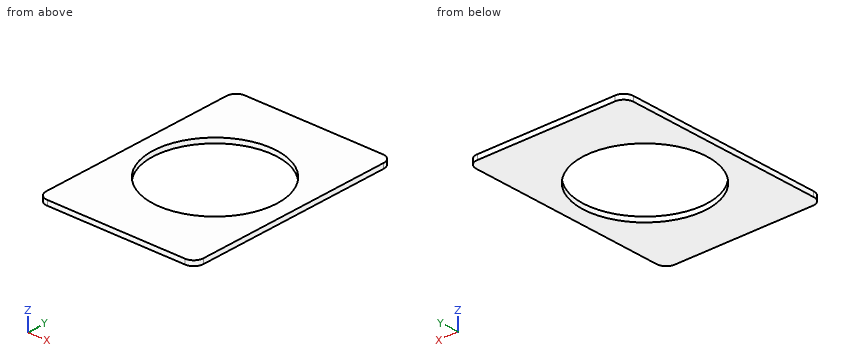
from build123d import *

# Parameters (mm, degrees)
F0_R     = 25
F1_DEPTH = 2


with BuildPart() as f1:
    # F0 (on Top) → F1 (new body)
    with BuildSketch(Plane.XY):
        with BuildLine():
            Line((31.70578804, -40.5199971151), (31.70578804, 40.5199971151))
            add(Edge.make_bspline(
                [(27.8376818991, 44.388103256), (29.9651402766, 44.388103256), (31.70578804, 42.6474554926), (31.70578804, 40.5199971151)],
                knots=[0, 0, 0, 0, 1, 1, 1, 1], degree=3))
            Line((27.8376818991, 44.388103256), (-27.8373296126, 44.388103256))
            add(Edge.make_bspline(
                [(-31.70578804, 40.5199971151), (-31.70578804, 42.6474554926), (-29.9651402766, 44.388103256), (-27.8373296126, 44.388103256)],
                knots=[0, 0, 0, 0, 1, 1, 1, 1], degree=3))
            Line((-31.70578804, 40.5199971151), (-31.70578804, -40.5199971151))
            add(Edge.make_bspline(
                [(-27.8373296126, -44.388103256), (-29.9651402766, -44.388103256), (-31.70578804, -42.6474554926), (-31.70578804, -40.5199971151)],
                knots=[0, 0, 0, 0, 1, 1, 1, 1], degree=3))
            Line((-27.8373296126, -44.388103256), (27.8376818991, -44.388103256))
            add(Edge.make_bspline(
                [(31.70578804, -40.5199971151), (31.70578804, -42.6474554926), (29.9651402766, -44.388103256), (27.8376818991, -44.388103256)],
                knots=[0, 0, 0, 0, 1, 1, 1, 1], degree=3))
        make_face()
        Circle(F0_R, mode=Mode.SUBTRACT)
    extrude(amount=F1_DEPTH)


solid = f1.part
CAD build for the part. Positions are in the model's coordinates, mm. Give positions to 0.01 mm unless a question says otherwise; leave off trailing zeros. Order: outer loops, then holes, each group sorted by start corner. A loop starts at its lowest first (then second) coordinate and runs counter-clockwise, first axis right, second up. Notation, with made-up numbers: (12, -34.75) - (22, -34.75) arc R7 ccw to (22, -24.75) - close; hole circle Ø5 at (8, 39). An arc over 180 degrees is marked (long way). Write each question's results on one line, items separated by ' | '.
1. Probe L1, parallel to Y at x = 0, z = 1.45; L2, parallel to X at y = 20, z = 1.8; L3, parallel to Y at x = 9.5, z = 0.55. List the from-to ranges inside material, lowest first. Write a range as from..to.
Calculated:
L1: y = -44.39..-25, 25..44.39 | L2: x = -31.71..-15, 15..31.71 | L3: y = -44.39..-23.12, 23.12..44.39
2. Saw through at A-A on x = 7. List the corners of the cut face in (y, z).
Calculated:
outline: (-44.39, 0) - (-24, 0) - (-24, 2) - (-44.39, 2) - close; (24, 0) - (44.39, 0) - (44.39, 2) - (24, 2) - close
3. Pin check, flat tip, straight feed: pin 1 (10 mm diameter, centred on x = -24, y = -4, fed in from +Z). Stop position of the tip, or through.
Calculated:
pin 1: stops at z = 2
4. Saw through at B-B on y = 0. List the corners of the cut face in (x, z).
Calculated:
outline: (-31.71, 0) - (-25, 0) - (-25, 2) - (-31.71, 2) - close; (25, 0) - (31.71, 0) - (31.71, 2) - (25, 2) - close
